from build123d import *

# Parameters (mm, degrees)
SKETCH1_R           = 1.375
BOSS_EXTRUDE1_DEPTH = 5
CUT_EXTRUDE1_DEPTH  = 3
SKETCH3_R           = 2.5
CUT_EXTRUDE2_DEPTH  = 2.5


with BuildPart() as part:
    # Sketch1 → Boss-Extrude1 (new body)
    with BuildSketch(Plane(origin=(0, 0, 0), x_dir=(1, 0, 0), z_dir=(0, 1, 0))):
        with BuildLine():
            Line((-40, -28.5), (40, -28.5))
            ThreePointArc((40, -28.5), (42.121320344, -27.621320344), (43, -25.5))
            Line((43, -25.5), (43, 25.5))
            ThreePointArc((43, 25.5), (42.121320344, 27.621320344), (40, 28.5))
            Line((40, 28.5), (-40, 28.5))
            ThreePointArc((-40, 28.5), (-42.121320344, 27.621320344), (-43, 25.5))
            Line((-43, 25.5), (-43, -25.5))
            ThreePointArc((-43, -25.5), (-42.121320344, -27.621320344), (-40, -28.5))
        make_face()
        with Locations(Location((0, 15, 0), (0, 0, 270))):
            Circle(SKETCH1_R, mode=Mode.SUBTRACT)
        with Locations(Location((-35, -15, 0), (0, 0, 270))):
            Circle(SKETCH1_R, mode=Mode.SUBTRACT)
        with Locations(Location((35, -15, 0), (0, 0, 270))):
            Circle(SKETCH1_R, mode=Mode.SUBTRACT)
        with Locations(Location((-39, 24.5, 0), (0, 0, 270))):
            Circle(SKETCH1_R, mode=Mode.SUBTRACT)
        with Locations(Location((19, 24.5, 0), (0, 0, 270))):
            Circle(SKETCH1_R, mode=Mode.SUBTRACT)
        with Locations(Location((19, -24.5, 0), (0, 0, 270))):
            Circle(SKETCH1_R, mode=Mode.SUBTRACT)
        with Locations(Location((-39, -24.5, 0), (0, 0, 270))):
            Circle(SKETCH1_R, mode=Mode.SUBTRACT)
        with BuildLine():
            Line((-37.052885882, 19.24229372), (-8.391974967, 15.448937863))
            ThreePointArc((-8.391974967, 15.448937863), (-7.147859594, 14.378709263), (-7.628511446, 12.809573795))
            Line((-7.628511446, 12.809573795), (-32.917550489, -8.264625407))
            ThreePointArc((-32.917550489, -8.264625407), (-34.421149889, -8.510435231), (-35.364225221, -7.313838997))
            Line((-35.364225221, -7.313838997), (-38.736097093, 17.553716061))
            ThreePointArc((-38.736097093, 17.553716061), (-38.312045905, 18.814232283), (-37.052885882, 19.24229372))
        make_face(mode=Mode.SUBTRACT)
        with BuildLine():
            Line((-1.577880073, 8.685099939), (-29.719509612, -14.76625801))
            ThreePointArc((-29.719509612, -14.76625801), (-29.964799607, -15.026060273), (-30.141686076, -15.33650443))
            Line((-30.141686076, -15.33650443), (-33.123332421, -22.4179145))
            ThreePointArc((-33.123332421, -22.4179145), (-32.990504952, -23.829720359), (-31.740879358, -24.5))
            Line((-31.740879358, -24.5), (11.772505288, -24.5))
            ThreePointArc((11.772505288, -24.5), (13.016699367, -23.83784312), (13.162424553, -22.435974791))
            Line((13.162424553, -22.435974791), (0.772315791, 8.096793229))
            ThreePointArc((0.772315791, 8.096793229), (-0.253358499, 8.987871314), (-1.577880073, 8.685099939))
        make_face(mode=Mode.SUBTRACT)
        with BuildLine():
            Line((-11.234499574, 24.5), (4.43151961, 24.5))
            ThreePointArc((4.43151961, 24.5), (5.913421136, 23.232309855), (4.890533381, 21.571957158))
            Line((4.890533381, 21.571957158), (0.321277785, 20.10326786))
            ThreePointArc((0.321277785, 20.10326786), (-0.003358772, 20.037341905), (-0.334549064, 20.044278553))
            Line((-0.334549064, 20.044278553), (-11.431312652, 21.512967851))
            ThreePointArc((-11.431312652, 21.512967851), (-12.7312541, 23.098619918), (-11.234499574, 24.5))
        make_face(mode=Mode.SUBTRACT)
        with BuildLine():
            Line((6.538594674, 15.494548288), (19, 19.5))
            Line((19, 19.5), (37.780665263, 24.865904361))
            ThreePointArc((37.780665263, 24.865904361), (39.177543611, 24.555066868), (39.678086712, 23.214415657))
            Line((39.678086712, 23.214415657), (35.10041997, -9.287018213))
            ThreePointArc((35.10041997, -9.287018213), (34.8636112, -9.909181999), (34.380888344, -10.367597546))
            Line((34.380888344, -10.367597546), (20.4998423, -18.609468634))
            ThreePointArc((20.4998423, -18.609468634), (19.255432614, -18.741284405), (18.344114904, -17.883711727))
            Line((18.344114904, -17.883711727), (5.607689179, 13.502480237))
            ThreePointArc((5.607689179, 13.502480237), (5.638666899, 14.70154708), (6.538594674, 15.494548288))
        make_face(mode=Mode.SUBTRACT)
        with BuildLine():
            Line((30.055567192, -22.022722512), (34.028332843, -20.397500201))
            ThreePointArc((34.028332843, -20.397500201), (34.927038281, -20.322741568), (35.706192222, -20.776811444))
            Line((35.706192222, -20.776811444), (37.51199479, -22.763194269))
            ThreePointArc((37.51199479, -22.763194269), (37.754252366, -24.421543548), (36.308517251, -25.269282328))
            Line((36.308517251, -25.269282328), (30.529949031, -24.908121814))
            ThreePointArc((30.529949031, -24.908121814), (29.14338695, -23.654387623), (30.055567192, -22.022722512))
        make_face(mode=Mode.SUBTRACT)
    extrude(amount=BOSS_EXTRUDE1_DEPTH)

    # Sketch2 → Cut-Extrude1 (cut)
    with BuildSketch(Plane(origin=(0, 5, 0), x_dir=(1, 0, 0), z_dir=(0, 1, 0))):
        Polygon((-36.113248654, 24.5), (-37.556624327, 27), (-40.443375673, 27), (-41.886751346, 24.5), (-40.443375673, 22), (-37.556624327, 22), align=None)
        Polygon((20.443375673, 27), (17.556624327, 27), (16.113248654, 24.5), (17.556624327, 22), (20.443375673, 22), (21.886751346, 24.5), align=None)
        Polygon((20.443375673, -22), (17.556624327, -22), (16.113248654, -24.5), (17.556624327, -27), (20.443375673, -27), (21.886751346, -24.5), align=None)
        Polygon((-36.113248654, -24.5), (-37.556624327, -22), (-40.443375673, -22), (-41.886751346, -24.5), (-40.443375673, -27), (-37.556624327, -27), align=None)
    extrude(amount=-CUT_EXTRUDE1_DEPTH, mode=Mode.SUBTRACT)

    # Sketch3 → Cut-Extrude2 (cut)
    with BuildSketch(Plane.XZ):
        with Locations(Location((-35, 15, 0), (0, 0, 270))):
            Circle(SKETCH3_R)
        with Locations(Location((35, 15, 0), (0, 0, 270))):
            Circle(SKETCH3_R)
        with Locations(Location((0, -15, 0), (0, 0, 270))):
            Circle(SKETCH3_R)
    extrude(amount=-CUT_EXTRUDE2_DEPTH, mode=Mode.SUBTRACT)


solid = part.part
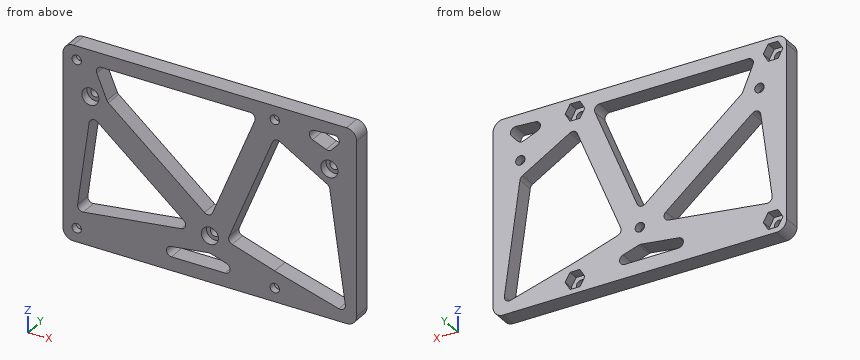
Work out the finished part from the listing and answer in its coordinate system (mm). Coordinates: 2 decimals unless noted, no trailing zeros. Loops run counter-clockwise (first coordinate to the right, second up) from the corner with the lowest first, then second, coordinate; pieces in that order, holes last. Notation, with made-up numbers: (84, 26.25) -> (110, 26.25) arc R24 cw to (110, 55.25) -> close; hole circle Ø10 at (11, 38). An arc over 180 degrees is marked (long way). Answer as CSV lines item,"result".
1) The part is cut by section A-A (z = 1). Give the vertices of the cut face in (x, y).
A:
outline,"(-43, 0) -> (-36.22, 0) -> (-36.22, 5) -> (-43, 5) -> close; (-24.2, 0) -> (-13.2, 0) -> (-13.2, 5) -> (-24.2, 5) -> close; (4.46, 0) -> (11.49, 0) -> (11.49, 5) -> (4.46, 5) -> close; (36.27, 0) -> (43, 0) -> (43, 5) -> (36.27, 5) -> close"
2) The part is cut by section B-B (x = -17.5). Give the vertices of the cut face in (y, z).
A:
outline,"(0, -28.5) -> (5, -28.5) -> (5, -16.65) -> (0, -16.65) -> close; (0, -4.58) -> (5, -4.58) -> (5, 4.58) -> (0, 4.58) -> close; (0, 24.5) -> (5, 24.5) -> (5, 28.5) -> (0, 28.5) -> close"
3) The part is cut by section C-C (y = 3.8). State how many separate pieces and enclosed holes the cut face has, and give its area (3 significant figures).
A:
separate pieces,"1"
enclosed holes,"12"
area,"2,350 mm²"
4) Straight lines are drawn through the part: probe 1 along Z at (x, y) = (-39, 1.35) (3 decimals); probe 2 along Z at (x, y) = (19, 1.4) (3 decimals); probe 3 along Z at (x, y) = (-2, 1.4). For each, find the intervals that lie inside material, in ascending order.
A:
probe 1,"z = -28.5 to -25.875, -23.125 to 23.125, 25.875 to 28.5"
probe 2,"z = -28.5 to -25.875, -23.125 to -19.5, 18.628 to 23.125, 25.875 to 28.5"
probe 3,"z = -28.5 to -24.5, -20.26 to -16.5, -13.5 to -8.33, 24.5 to 28.5"
5) A flat-ended cylindrical pin translates along its axis: pin 1 (2.5 mm diameter, centred on x = -34, z = 15.5, fed in from -Y). Find the tip coordinate at first contact, or state that the pin passes through.
A:
pin 1,"stops at y = 2.5"
